```python
from build123d import *

# Parameters (mm, degrees)
F1_DEPTH = 38.1
F2_DEPTH = 25.4


with BuildPart() as f1:
    # F0 (on Front) → F1 (new body)
    with BuildSketch(Plane.XZ):
        Polygon((25.092965, -4.49749), (-16.305355, 35.833862), (-57.258341, 35.833862), (-57.258341, -35.833862), (57.258341, -35.833862), align=None)
    extrude(amount=F1_DEPTH)

    # F0 (on Front) → F2 (join)
    with BuildSketch(Plane.XZ):
        Polygon((57.258341, -4.49749), (25.092965, -4.49749), (57.258341, -35.833862), align=None)
    extrude(amount=F2_DEPTH)


solid = f1.part
```
Model file for the job. Use its own axes, mm. A direction names the side the tool comes from. Round coordinates to 2 decimals unless told otherwise and drop trailing zeros. Write each loop counter-clockwise with the first axis right and the second up, starting at its lowest first coordinate (ties: lowest second). Pieces come first, ordered by that corner, then holes. Notation, with made-up numbers: (57, 78) - (105, 78) arc R30 cw to (105, 106) - close; hole circle Ø4 at (-25, 49.25). An arc over 180 degrees is marked (long way). One line per item, written item: value.
(1) Drop flat-ended pins along their axis: P1, Ø8, axis at x = 24, y = -10.5, coming from the +Z side; P2, Ø20.5, axis at x = 42.5, y = -18, coming from the +Z side; P3, Ø1.5, axis at y = -27, z = 26.5, coming from the +X side. Give the stop position or say it passes through.
Values follow:
P1: stops at z = 0.46
P2: stops at z = -4.5
P3: stops at x = -5.95
(2) Cut at B-B, the plane z = -9. Give the cut face in (x, y), plus the area to 3 significant figures.
Values follow:
outline: (-57.26, -38.1) - (29.71, -38.1) - (29.71, -25.4) - (57.26, -25.4) - (57.26, 0) - (-57.26, 0) - close
area: 4,010 mm²
(3) 3-axis set-ups, long thin cutter, end or side, ignore diameter. For faces 1 (the flat face through (57.258, -13, -20)), 2 (the flat face through (41, -13, -4.497)), 3 (the flat face through (48, -25.4, -13)): which of +Z, -Z, +X, -X, +Y, -Y reach the whole face in a straight line?
Values follow:
face 1: +Z, -Z, +X, +Y, -Y
face 2: +Z, +X, +Y, -Y
face 3: +Z, +X, -Y
(4) Cut at C-C, the plane y = -6. Give the cut face in (x, z).
Values follow:
outline: (-57.26, -35.83) - (57.26, -35.83) - (57.26, -4.5) - (25.09, -4.5) - (-16.31, 35.83) - (-57.26, 35.83) - close
(5) Cut at A-A, the plane y = -31. Give the cut face in (x, z).
Values follow:
outline: (-57.26, -35.83) - (57.26, -35.83) - (-16.31, 35.83) - (-57.26, 35.83) - close
(6) Wall check: probe 1 along Z at (x, y) = (52, -16); probe 2 along Y at (x, z) = (49.5, -20.5); probe 3 along Z at (x, y) = (0.5, -27). Give the ranges that are in metal, low to high.
Values follow:
probe 1: z = -35.83 to -4.5
probe 2: y = -25.4 to 0
probe 3: z = -35.83 to 19.46
(7) Cut at D-D, the plane x = 6. Give the cut face in (y, z).
Values follow:
outline: (-38.1, -35.83) - (0, -35.83) - (0, 14.1) - (-38.1, 14.1) - close
